from build123d import *

# Parameters (mm, degrees)
SKETCH_1_W          = 20
SKETCH_1_H          = 9.5
EXTRUDE_1_DEPTH     = 47
SKETCH_2_W          = 47
SKETCH_2_H          = 20
SKETCH_2_H_2        = 4
EXTRUDE_2_DEPTH     = 8.5
SKETCH_3_R          = 2
CUT_EXTRUDE_1_DEPTH = 8.5


with BuildPart() as part:
    # 草图1 → 凸台-拉伸1 (new body)
    with BuildSketch(Plane(origin=(0, 0, 0), x_dir=(0, 0, -1), z_dir=(1, 0, 0))):
        Rectangle(SKETCH_1_W, SKETCH_1_H)
    extrude(amount=EXTRUDE_1_DEPTH)

    # 草图2 → 凸台-拉伸2 (add)
    with BuildSketch(Plane(origin=(0, 4.75, 0), x_dir=(1, 0, 0), z_dir=(0, 1, 0))):
        with Locations((23.5, 0)):
            Rectangle(SKETCH_2_W, SKETCH_2_H)
        with Locations((23.5, 12)):
            Rectangle(SKETCH_2_W, SKETCH_2_H_2)
        with Locations((23.5, -12)):
            Rectangle(SKETCH_2_W, SKETCH_2_H_2)
    extrude(amount=EXTRUDE_2_DEPTH)

    # 草图3 → 切除-拉伸1 (cut)
    with BuildSketch(Plane(origin=(0, 13.25, 0), x_dir=(1, 0, 0), z_dir=(0, 1, 0))):
        with Locations(Location((14.25, 9.25, 0), (0, 0, 270))):
            Circle(SKETCH_3_R)
        with Locations(Location((32.75, 9.25, 0), (0, 0, 22.024312837))):
            Circle(SKETCH_3_R)
        with Locations(Location((32.75, -9.25, 0), (0, 0, 270))):
            Circle(SKETCH_3_R)
        with Locations(Location((14.25, -9.25, 0), (0, 0, 337.975687163))):
            Circle(SKETCH_3_R)
    extrude(amount=-CUT_EXTRUDE_1_DEPTH, mode=Mode.SUBTRACT)


solid = part.part
Check sheet for the modelled part. Datum: model origin and axes. Units: mm. A direction names the side the tool comes from. Give positions to 0.01 mm unless a question says otherwise; leave off trailing zeros. Write each loop counter-clockwise with the first axis right and the second up, starting at its lowest first coordinate (ties: lowest second). Pieces come first, ordered by that corner, then holes. Notation, with made-up numbers: (1.25, 73.25) -> (39.25, 73.25) arc R10 cw to (39.25, 79.25) -> close; hole circle Ø6 at (-31.5, 43.5). An arc over 180 degrees is marked (long way). Write item = value, one per line.
Item 1: Sectioned sample at B-B on z = 9.25. Record the boundary of the cut face in (x, y).
Output:
outline = (0, -4.75) -> (47, -4.75) -> (47, 13.25) -> (34.75, 13.25) -> (34.75, 4.75) -> (30.75, 4.75) -> (30.75, 13.25) -> (16.25, 13.25) -> (16.25, 4.75) -> (12.25, 4.75) -> (12.25, 13.25) -> (0, 13.25) -> close
Item 2: Sectioned sample at D-D on y = -2.75. Record the boundary of the cut face in (x, z), and give its area (3 significant figures).
Output:
outline = (0, -10) -> (47, -10) -> (47, 10) -> (0, 10) -> close
area = 940 mm^2
Item 3: Sectioned sample at C-C on y = 9.75. Record the boundary of the cut face in (x, z), and give its area (3 significant figures).
Output:
outline = (0, -14) -> (47, -14) -> (47, 14) -> (0, 14) -> close; hole circle Ø4 at (14.25, -9.25); hole circle Ø4 at (14.25, 9.25); hole circle Ø4 at (32.75, -9.25); hole circle Ø4 at (32.75, 9.25)
area = 1,270 mm^2
Item 4: Gauge pin test, flat ends, axial feed: pin 1 (2 mm diameter, centred on x = 24.5, y = 1, fed in from +Z); pin 2 (2 mm diameter, centred on x = 33.5, z = 9, fed in from +Y); pin 3 (2 mm diameter, centred on x = 31, z = -11.5, fed in from -Y). Record the tip position at first contact, or that the pin passes through.
Output:
pin_1 = 10
pin_2 = 4.75
pin_3 = 4.75
Item 5: Tool access check on faces 4 (the flat face through (23, 0, 10)), 5 (the flat face through (33, 4.75, -9)), 6 (the flat face through (23, 13.25, 0)), 7 (the flat face through (23, 4.75, -12)), 8 (the flat face through (23, 9, 14)). Record the directions out of +Z, -Z, +X, -X, +Y, -Y that give a thin tool (end or side, any length) a straight path to the whole face; none if there is none.
Output:
face_4 = +Z, +X, -X, -Y
face_5 = +Y
face_6 = +Z, -Z, +X, -X, +Y
face_7 = -Z, +X, -X, -Y
face_8 = +Z, +X, -X, +Y, -Y
Item 6: Scan lines: probe 1 along X at (y, z) = (11.5, -9.25); probe 2 along Z at (x, y) = (32.75, 7); probe 3 along Z at (x, y) = (16, 8). Record each from-to range of solid material in increasing order. Write a range as from..to.
Output:
probe_1 = 0..12.25, 16.25..30.75, 34.75..47
probe_2 = -14..-11.25, -7.25..7.25, 11.25..14
probe_3 = -14..-10.22, -8.28..8.28, 10.22..14
Item 7: Release check for a two-part mould opening along X. For faces 1 (the flat face through (0, 4, 0)), 2 (the cylindrical face through (16.244, 9.06, 9.408)), 3 (the flat face through (23, 0, -10)) record: +X half, -X half, draft (parallel to the pull), parting line (faces both ways), or undercut.
Output:
face_1 = -X half
face_2 = undercut
face_3 = draft
Item 8: Sectioned sample at A-A on x = 14.25. Record the boundary of the cut face in (y, z), and give its area (3 significant figures).
Output:
outline = (-4.75, -10) -> (4.75, -10) -> (4.75, -7.25) -> (13.25, -7.25) -> (13.25, 7.25) -> (4.75, 7.25) -> (4.75, 10) -> (-4.75, 10) -> close; (4.75, -14) -> (13.25, -14) -> (13.25, -11.25) -> (4.75, -11.25) -> close; (4.75, 11.25) -> (13.25, 11.25) -> (13.25, 14) -> (4.75, 14) -> close
area = 360 mm^2
